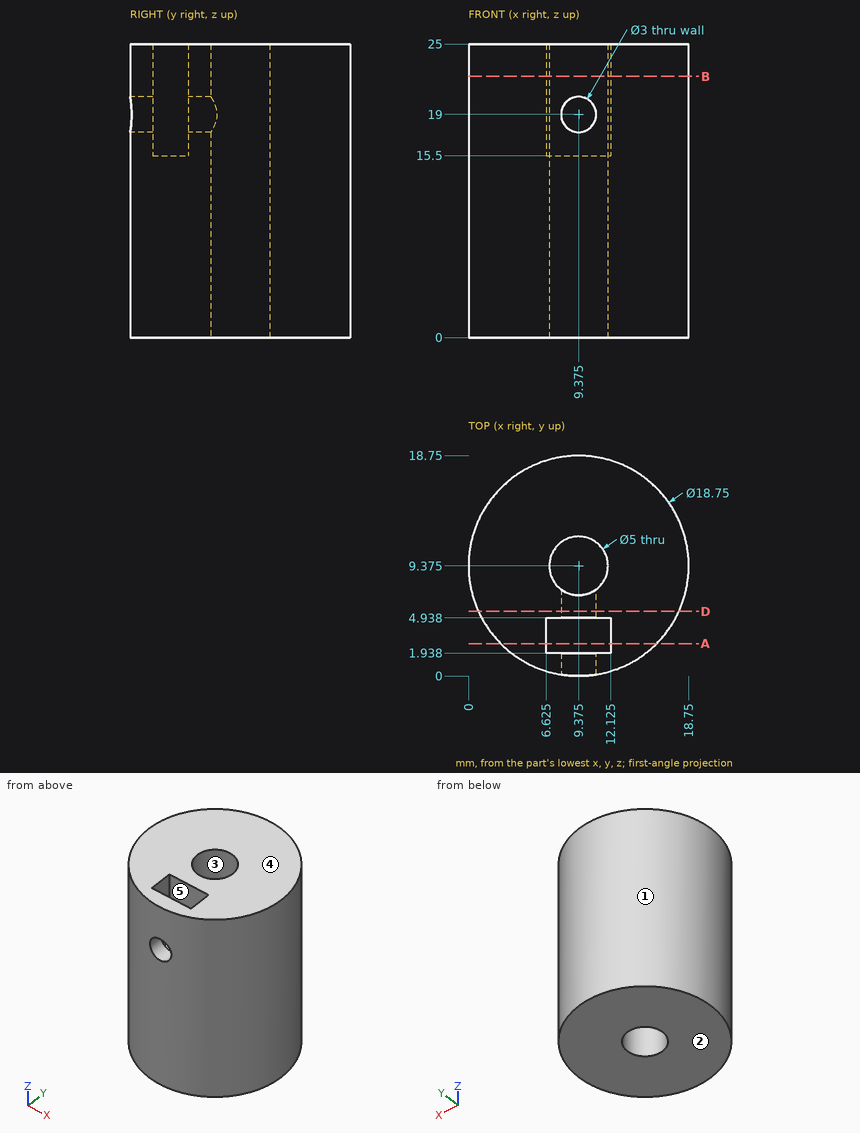
Geometry: see drawing. Coordinates: mm, zero at the bounding-box minimum. A direction names the side the tool comes from. Give positions to 0.01 mm unless a question says otherwise; leave off trailing zeros. Loops run counter-clockwise (first coordinate to the right, second up) from the corner with the lowest first, then second, coordinate; pieces in that order, holes last. Notation, with made-up numbers: (0, 47) - (15, 47) arc R24 cw to (15, 61) - close; hole circle Ø3 at (16.5, 78.25). An arc over 180 degrees is marked (long way). Use CSV: the item, a comma, the result in double quotes. Start each with the question number.
Item 1: Mould query, pull axis Y, two halves, no side actions, for the marked faces 1, 2 and 3. Classes: pulls with the +Y half, pulls with the -Y half, needs draft (parallel to the pull), parting line crosses it, or undercut.
Item 2: Reachability of the marked faces 4 and 5 from +Z, -Z, +X, -X, +Y, -Y: full face, straight path, thin tool, end or side. Return the list, or none.
Item 3: Section D-D on y = 5.5. Return loops of the section in (x, z) (1 decimal), then the cut area to 3 significant figures.
Item 4: Contact query for flat-ended pins moving along their axis: P1, Ø0.9, axis at y = 3, z = 22, coming from the +X side; P2, Ø4, axis at x = 15, z = 7, coming from the +Y side; P3, Ø6, axis at y = 16.5, z = 17, coming from the +X side. Output: stop coordinate, or through.
Item 5: Section B-B on z = 22.25. State how many separate pieces and enclosed holes the cut face has, then the cut area to 3 significant figures.
Item 6: Line query: line 1 (Y direction, x = 11, z = 18) (1 decimal); line 2 (X direction, y = 4.75, z = 23.75) (1 decimal); line 3 (X direction, y = 10.5, z = 15.25). Output: solid intervals per line, ascending.
Item 7: Section A-A on y = 2.75. Return loops of the section in (x, z) (1 decimal).
Ans:
1,face 1,"parting line crosses it"
1,face 2,"needs draft"
1,face 3,"undercut"
2,face 4,"+Z, +X, -X, +Y, -Y"
2,face 5,"+Z"
3,outline,"(0.8, 0) - (17.9, 0) - (17.9, 25) - (0.8, 25) - close; hole circle Ø3 at (9.4, 19)"
3,area,"420 mm2"
4,P1,"stops at x = 16.64"
4,P2,"stops at y = 18.02"
4,P3,"stops at x = 17.79"
5,separate pieces,"1"
5,enclosed holes,"2"
5,area,"240 mm2"
6,line 1,"y = 0.1 to 1.9, 4.9 to 7.5, 11.3 to 18.6"
6,line 2,"x = 1.2 to 6.6, 12.1 to 17.5"
6,line 3,"x = 0.07 to 7.14, 11.61 to 18.68"
7,outline,"(2.7, 0) - (16, 0) - (16, 25) - (12.1, 25) - (12.1, 15.5) - (6.6, 15.5) - (6.6, 25) - (2.7, 25) - close"
